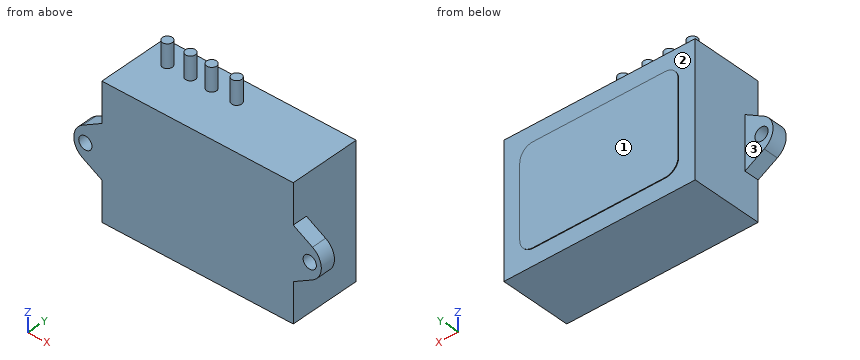
from build123d import *

# Parameters (mm, degrees)
SKETCH1_W           = 58
SKETCH1_H           = 40
BOSS_EXTRUDE1_DEPTH = 21.5
BOSS_EXTRUDE2_DEPTH = 4.5
SKETCH3_R           = 2
CUT_EXTRUDE1_DEPTH  = 80.443376061
BOSS_EXTRUDE3_DEPTH = 0.2
SKETCH6_R           = 1.5
BOSS_EXTRUDE4_DEPTH = 7
SKETCH8_R           = 1.5
BOSS_EXTRUDE6_DEPTH = 7
SKETCH9_R           = 1.5
BOSS_EXTRUDE7_DEPTH = 7


with BuildPart() as part:
    # Sketch1 → Boss-Extrude1 (new body)
    with BuildSketch(Plane(origin=(0, 0, 0), x_dir=(1, 0, 0), z_dir=(0, 1, 0))):
        with Locations((29, 20)):
            Rectangle(SKETCH1_W, SKETCH1_H)
    extrude(amount=BOSS_EXTRUDE1_DEPTH)

    # Sketch2 → Boss-Extrude2 (add)
    with BuildSketch(Plane(origin=(0, 0, 0), x_dir=(1, 0, 0), z_dir=(0, 1, 0))):
        with BuildLine():
            Line((0, 28), (0, 12))
            Line((0, 12), (-5.82179677, 15.361215932))
            ThreePointArc((-5.82179677, 15.361215932), (-8.5, 20), (-5.82179677, 24.638784068))
            Line((-5.82179677, 24.638784068), (0, 28))
        make_face()
        with BuildLine():
            Line((58, 28), (63.82179677, 24.638784068))
            ThreePointArc((63.82179677, 24.638784068), (66.5, 20), (63.82179677, 15.361215932))
            Line((63.82179677, 15.361215932), (58, 12))
            Line((58, 12), (58, 28))
        make_face()
    extrude(amount=BOSS_EXTRUDE2_DEPTH)

    # Sketch3 → Cut-Extrude1 (cut, through all)
    with BuildSketch(Plane(origin=(0, 4.5, 0), x_dir=(1, 0, 0), z_dir=(0, 1, 0))):
        with Locations(Location((-5, 20, 0), (0, 0, 270))):
            Circle(SKETCH3_R)
        with Locations(Location((63, 20, 0), (0, 0, 90))):
            Circle(SKETCH3_R)
    extrude(amount=-CUT_EXTRUDE1_DEPTH, mode=Mode.SUBTRACT)

    # Sketch4 → Boss-Extrude3 (add)
    with BuildSketch(Plane(origin=(0, 21.5, 0), x_dir=(1, 0, 0), z_dir=(0, 1, 0))):
        with BuildLine():
            Line((5, 31), (5, 9))
            ThreePointArc((5, 9), (6.171572875, 6.171572875), (9, 5))
            Line((9, 5), (49, 5))
            ThreePointArc((49, 5), (51.828427125, 6.171572875), (53, 9))
            Line((53, 9), (53, 31))
            ThreePointArc((53, 31), (51.828427125, 33.828427125), (49, 35))
            Line((49, 35), (9, 35))
            ThreePointArc((9, 35), (6.171572875, 33.828427125), (5, 31))
        make_face()
    extrude(amount=BOSS_EXTRUDE3_DEPTH)

    # Sketch6 → Boss-Extrude4 (add)
    with BuildSketch(Plane.XY):
        with Locations((7, 14.5)):
            Circle(SKETCH6_R)
    extrude(amount=BOSS_EXTRUDE4_DEPTH)

    # Sketch8 → Boss-Extrude6 (add)
    with BuildSketch(Plane.XY):
        with Locations(Location((14, 14.5, 0), (0, 0, 180))):
            Circle(SKETCH8_R)
        with Locations(Location((28, 14.5, 0), (0, 0, 180))):
            Circle(SKETCH8_R)
    extrude(amount=BOSS_EXTRUDE6_DEPTH)

    # Sketch9 → Boss-Extrude7 (add)
    with BuildSketch(Plane.XY):
        with Locations(Location((20.412696723, 14.5, 0), (0, 0, 180))):
            Circle(SKETCH9_R)
    extrude(amount=BOSS_EXTRUDE7_DEPTH)


solid = part.part
Check sheet for the modelled part. Datum: model origin and axes. Units: mm. Face numbers are marked on the shaded views. A direction names the side the tool comes from. Round coordinates to 2 decimals unless told otherwise and drop trailing zeros. Loops run counter-clockwise (first coordinate to the right, second up) from the corner with the lowest first, then second, coordinate; pieces in that order, holes last.
1. Gauge pin test, flat ends, axial feed: pin 1 Ø1.5 at (x, y) = (20, 4.5) entering from +Z; pin 2 Ø2.5 at (x, z) = (-4, -23.5) entering from +Y; pin 3 Ø3 at (x, z) = (-5, -20) entering from +Y; pin 4 Ø12 at (y, z) = (19, -24) entering from +X. Record the tip position at first contact, or that the pin passes through.
2. Sectioned sample at D-D on y = 7. Record the boundary of the cut face in (x, z), and give its area (3 significant figures).
3. Scan lines: probe 1 along X at (y, z) = (5.5, -9.5); probe 2 along Z at (x, y) = (11.5, 16.5); probe 3 along Y at (x, z) = (52, -4.5). Record each from-to range of solid material in increasing order.
4. Set-up check for the marked faces 1, 2 and 3: record each of +Z, -Z, +X, -X, +Y, -Y from which the full face is reachable in a straight line by a thin tool's end or side.
5. Sectioned sample at C-C on x = 33. Record the boundary of the cut face in (y, z), and give its area (3 significant figures).
6. Sectioned sample at B-B on x = -5. Record the boundary of the cut face in (y, z), and give its area (3 significant figures).
7. Sectioned sample at A-A on z = -20. Record the boundary of the cut face in (x, y), and give its area (3 significant figures).
Recorded:
1. pin 1: stops at z = 0
1. pin 2: stops at y = 4.5
1. pin 3: passes through
1. pin 4: stops at x = 58
2. outline: (0, -40) - (58, -40) - (58, 0) - (0, 0) - close
2. area: 2,320 mm2
3. probe 1: x = 0 to 58
3. probe 2: z = -40 to 0
3. probe 3: y = 0 to 21.5
4. face 1: +Z, -Z, +X, -X, +Y
4. face 2: +Y
4. face 3: +Z, -Z, -X, +Y
5. outline: (0, -40) - (21.5, -40) - (21.5, -35) - (21.7, -35) - (21.7, -5) - (21.5, -5) - (21.5, 0) - (0, 0) - close
5. area: 866 mm2
6. outline: (0, -25.11) - (4.5, -25.11) - (4.5, -22) - (0, -22) - close; (0, -18) - (4.5, -18) - (4.5, -14.89) - (0, -14.89) - close
6. area: 28.0 mm2
7. outline: (-8.5, 0) - (-7, 0) - (-7, 4.5) - (-8.5, 4.5) - close; (-3, 0) - (61, 0) - (61, 4.5) - (58, 4.5) - (58, 21.5) - (53, 21.5) - (53, 21.7) - (5, 21.7) - (5, 21.5) - (0, 21.5) - (0, 4.5) - (-3, 4.5) - close; (65, 0) - (66.5, 0) - (66.5, 4.5) - (65, 4.5) - close
7. area: 1,300 mm2
